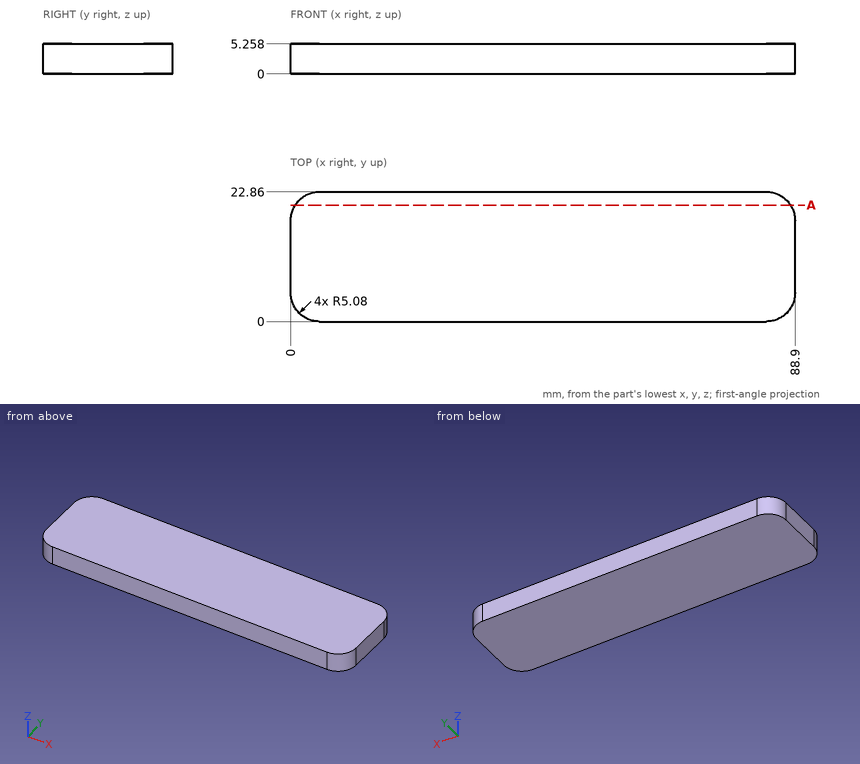
The figure shows three views and two pictorial views of one solid part (mm, origin at its lowest corner). Answer the questions. Coordinates: 2 decimals unless noted, no trailing zeros. Loops run counter-clockwise (first coordinate to the right, second up) from the corner with the lowest first, then second, coordinate; pieces in that order, holes last. Notation, with made-up numbers: (85, 65) -> (111, 65) arc R21 cw to (111, 100) -> close; hole circle Ø6 at (12.5, 79). An arc over 180 degrees is marked (long way). Write item = value, one per line. Start each with the question number.
1) Given pin 1 Ø2 at (y, z) = (3, 2.5) entering from +X, flat-ended and moving along its own axis, determine where the tip first touches the part or whether it passes through.
2) A cutting plane is placed at A-A (y = 20.5). Give the vertices of the cut face in (x, z), then the cut area to 3 significant figures.
3) Straight lines are drawn through the part: line 1 (X direction, y = 18, z = 1.85) (1 decimal); line 2 (X direction, y = 18.5, z = 4.4). For each, find the intervals that lie inside material, in ascending order. Write a range as from..to.
Responses:
q1.pin_1 = 88.78
q2.outline = (0.79, 0) -> (88.11, 0) -> (88.11, 5.26) -> (0.79, 5.26) -> close
q2.area = 459 mm²
q3.line_1 = 0..88.9
q3.line_2 = 0.05..88.85
